For this review, take the finished solid that the model builds, in its own axes (mm). A direction names the side the tool comes from. Give positions to 0.01 mm unless a question says otherwise; leave off trailing zeros. Loops run counter-clockwise (first coordinate to the right, second up) from the corner with the lowest first, then second, coordinate; pieces in that order, holes last. Notation, with made-up numbers: (0.25, 11) - (37.25, 11) arc R27 ccw to (37.25, 36) - close; hole circle Ø6 at (18, 4). An arc over 180 degrees is marked (long way). Answer as CSV lines item,"result".
from build123d import *

# Parameters (mm, degrees)
SKETCH_2_W          = 15.902311404
SKETCH_2_H          = 11.3
EXTRUDE_1_DEPTH     = 5
EXTRUDE_2_DEPTH     = 1
EXTRUDE_4_DEPTH     = 1
SKETCH_6_W          = 15.902311404
SKETCH_6_H          = 11.3
CUT_EXTRUDE_1_DEPTH = 36.003849734
SKETCH_7_W          = 27.70005588
SKETCH_7_H          = 1.6
CUT_EXTRUDE_2_DEPTH = 6
EXTRUDE_5_DEPTH     = 84.1
SKETCH_9_W          = 32
SKETCH_9_H          = 4.6
EXTRUDE_6_DEPTH     = 2
SKETCH_10_W         = 11.391343663
SKETCH_10_H         = 5.9
CUT_EXTRUDE_3_DEPTH = 6


with BuildPart() as part:
    # 草图2 → 凸台-拉伸1 (new body)
    with BuildSketch(Plane.XY):
        Polygon((-1.806344933, -3), (28.193655067, -3), (28.193655067, 17), (10.291343663, 17), (10.291343663, 9.5), (-1.806344933, 9.5), align=None)
        with Locations((19.242499365, 7.25)):
            Rectangle(SKETCH_2_W, SKETCH_2_H, mode=Mode.SUBTRACT)
    extrude(amount=EXTRUDE_1_DEPTH)

    # 草图3 → 凸台-拉伸2 (add)
    with BuildSketch(Plane.XY.offset(5)):
        Polygon((-2.806344933, -3), (29.193655067, -3), (29.193655067, 18), (9.291343663, 18), (9.291343663, 10.5), (-2.806344933, 10.5), align=None)
    extrude(amount=EXTRUDE_2_DEPTH)

    # 草图5 → 凸台-拉伸4 (add)
    with BuildSketch(Plane(origin=(0, 0, 0), x_dir=(-1, 0, 0), z_dir=(0, 0, -1))):
        Polygon((-29.193655067, 18), (-29.193655067, -3), (-28.193655067, -3), (1.806344933, -3), (2.806344933, -3), (2.806344933, 10.5), (-9.291343663, 10.5), (-9.291343663, 18), align=None)
    extrude(amount=EXTRUDE_4_DEPTH)

    # 草图6 → 切除-拉伸1 (cut, through all)
    with BuildSketch(Plane.XY.offset(6)):
        with Locations((19.242499365, 7.25)):
            Rectangle(SKETCH_6_W, SKETCH_6_H)
    extrude(amount=-CUT_EXTRUDE_1_DEPTH, mode=Mode.SUBTRACT)

    # 草图7 → 切除-拉伸2 (cut)
    with BuildSketch(Plane(origin=(0, 0, -1), x_dir=(-1, 0, 0), z_dir=(0, 0, -1))):
        with Locations((-13.75002794, 0.8)):
            Rectangle(SKETCH_7_W, SKETCH_7_H)
    extrude(amount=-CUT_EXTRUDE_2_DEPTH, mode=Mode.SUBTRACT)

    # 草图8 → 凸台-拉伸5 (add)
    with BuildSketch(Plane(origin=(0, 0, -1), x_dir=(-1, 0, 0), z_dir=(0, 0, -1))):
        Polygon((-27.60005588, 1.6), (-29.193655067, 1.6), (-29.193655067, -3), (2.806344933, -3), (2.806344933, 1.6), (0.1, 1.6), (0.1, 0), (-27.60005588, 0), align=None)
    extrude(amount=EXTRUDE_5_DEPTH)

    # 草图9 → 凸台-拉伸6 (add)
    with BuildSketch(Plane(origin=(0, 0, -85.1), x_dir=(-1, 0, 0), z_dir=(0, 0, -1))):
        with Locations((-13.193655067, -0.7)):
            Rectangle(SKETCH_9_W, SKETCH_9_H)
    extrude(amount=EXTRUDE_6_DEPTH)

    # 草图10 → 切除-拉伸3 (cut)
    with BuildSketch(Plane(origin=(0, 0, -1), x_dir=(-1, 0, 0), z_dir=(0, 0, -1))):
        with Locations((-5.595671832, 4.55)):
            Rectangle(SKETCH_10_W, SKETCH_10_H)
    extrude(amount=-CUT_EXTRUDE_3_DEPTH, mode=Mode.SUBTRACT)


solid = part.part
1) Wall thickness on line 1 (Y direction, x = 5, z = -76); line 2 (Z direction, x = 22.5, y = 14); line 3 (Z direction, x = 0, y = 3.25): over which ranges is each line inside the solid? List them lowest first. Write a range as from..to.
From the geometry:
line 1,"y = -3..0"
line 2,"z = -1..6"
line 3,"z = 5..6"
2) Consider section B-B on x = 22. Write out the cut boundary in (y, z).
From the geometry:
outline,"(-3, -87.1) - (1.6, -87.1) - (1.6, -85.1) - (0, -85.1) - (0, 5) - (1.6, 5) - (1.6, 6) - (-3, 6) - close; (12.9, -1) - (18, -1) - (18, 0) - (17, 0) - (17, 5) - (18, 5) - (18, 6) - (12.9, 6) - close"
3) Consider section D-D on x = 3. Write out the cut boundary in (y, z).
From the geometry:
outline,"(-3, -87.1) - (1.6, -87.1) - (1.6, -85.1) - (0, -85.1) - (0, 5) - (7.5, 5) - (7.5, -1) - (10.5, -1) - (10.5, 0) - (9.5, 0) - (9.5, 5) - (10.5, 5) - (10.5, 6) - (-3, 6) - close"
4) Consider section A-A on y = 11.75. Write out the cut boundary in (x, z), and give its area (3 significant figures).
From the geometry:
outline,"(9.29, -1) - (11.29, -1) - (11.29, 6) - (9.29, 6) - (9.29, 5) - (10.29, 5) - (10.29, 0) - (9.29, 0) - close; (27.19, -1) - (29.19, -1) - (29.19, 0) - (28.19, 0) - (28.19, 5) - (29.19, 5) - (29.19, 6) - (27.19, 6) - close"
area,"18.0 mm^2"
5) Insertion check: P1, Ø2, axis at x = 5.5, z = -13, coming from the +Y side; P2, Ø4, axis at y = 2.5, z = 2.5, coming from the +X side; P3, Ø2, axis at y = 3.5, z = -52.5, coming from the +X side; P4, Ø2.5, axis at y = 1.5, z = 1.5, coming from the -X side. Each pin has a flat end and moves straight along its axis. Give the tip position at first contact, or say it passes through.
From the geometry:
P1,"stops at y = 0"
P2,"stops at x = 28.19"
P3,"passes through"
P4,"stops at x = -1.81"
6) Machinability: for faces 4 (the flat face through (-1.806, 3, 2)), 5 (the flat face through (10, 10, 0)), 6 (the flat face through (28.194, 7, 2)), which of the approach directions +Z, -Z, +X, -X, +Y, -Y give a long, thin tool a straight path to every point of the face, cutting with its end or side? Answer none if there is none.
From the geometry:
face 4,"-X, +Y, -Y"
face 5,"+Y"
face 6,"+X, +Y, -Y"
7) Draft analysis for pull direction Z (two halves, no side actions). For faces 1 (the flat face through (13, -1, -87.1)), 2 (the flat face through (4, 9.5, 2)), 3 (the flat face through (11.291, 10, 3)), state which applies: pulls with the +Z half, pulls with the -Z half, needs draft (parallel to the pull), parting line crosses it, or undercut.
From the geometry:
face 1,"pulls with the -Z half"
face 2,"undercut"
face 3,"needs draft"
8) Consider section C-C on y = 4.5. Write out the cut boundary in (x, z).
From the geometry:
outline,"(-2.81, -1) - (-0.1, -1) - (-0.1, 5) - (11.29, 5) - (11.29, 6) - (-2.81, 6) - (-2.81, 5) - (-1.81, 5) - (-1.81, 0) - (-2.81, 0) - close; (27.19, -1) - (29.19, -1) - (29.19, 0) - (28.19, 0) - (28.19, 5) - (29.19, 5) - (29.19, 6) - (27.19, 6) - close"
